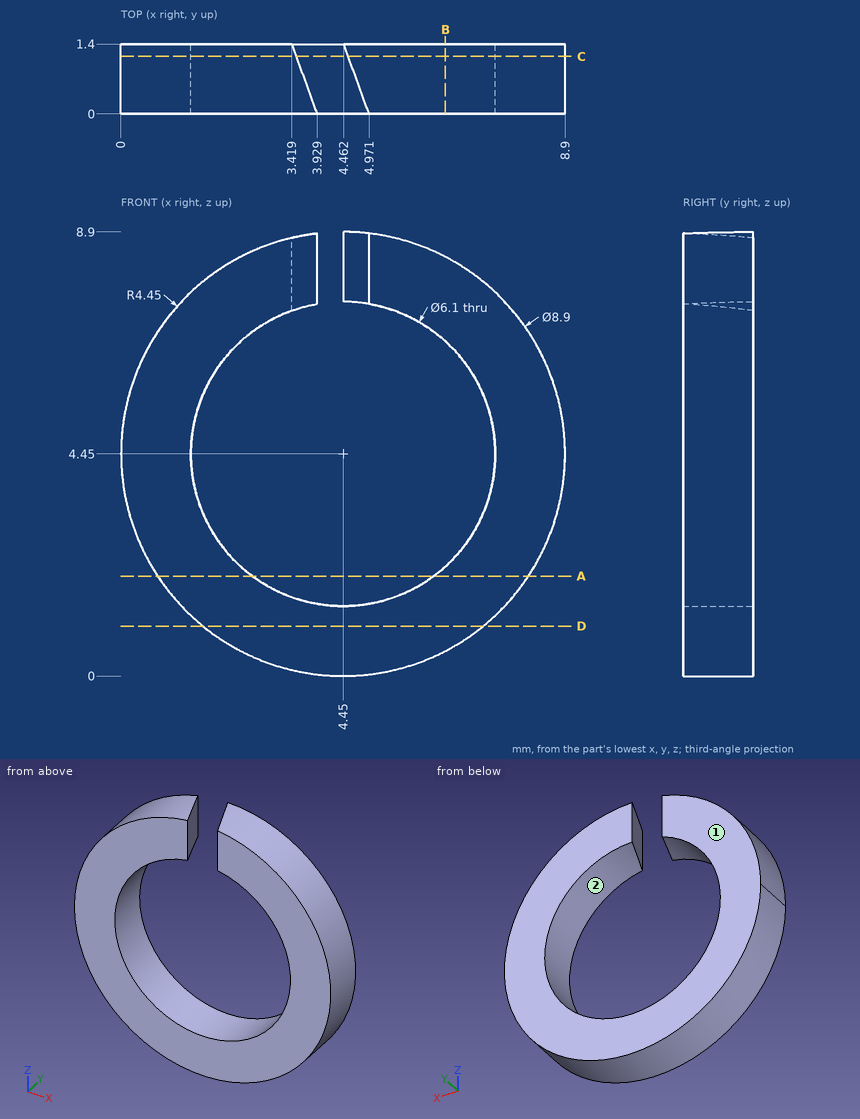
Design review of the part shown in the three views and the two pictorial views. Dimensions are in mm from the part's minimum x, y and z. Coordinates: 2 decimals unless noted, no trailing zeros. Order: outer loops, then holes, each group sorted by start corner. A loop starts at its lowest first (then second) coordinate and runs counter-clockwise, first axis right, second up.
1) Clearance check with flat-ended pins moving along their axes: pin 1 (3 mm diameter, centred on x = 8, z = 7.5, fed in from -Y); pin 2 (5 mm diameter, centred on x = 4.45, z = 4.45, fed in from -Y). State where each tip first meets the part, or that it passes through.
2) Mouldability with a two-part tool opening along X and no side actions: class the marked faces 1 and 2 as +X half, -X half, draft (parallel to the pull), parting line (faces both ways), or undercut.
3) Take a section at A-A, the plane z = 2. Give the boundary of the cut face in (x, y) (1 decimal).
4) Wall thickness on line 1 along X through (y, z) = (0.6, 4.5); line 2 along Z through (x, y) = (4.45, 1.05); line 3 along X through (y, z) = (1.3, 3.5): over which ranges is each line inside the solid? List them lowest first.
5) Take a section at C-C, the plane y = 1.15. Give the boundary of the cut face in (x, z).
6) Take a section at B-B, the plane x = 6.5. Give the boundary of the cut face in (y, z).
7) Take a section at D-D, the plane z = 1. Give the boundary of the cut face in (x, y).
Returned:
1. pin 1: stops at y = 0
1. pin 2: passes through
2. face 1: draft
2. face 2: undercut
3. outline: (0.7, 0) - (2.6, 0) - (2.6, 1.4) - (0.7, 1.4) - close; (6.3, 0) - (8.2, 0) - (8.2, 1.4) - (6.3, 1.4) - close
4. line 1: x = 0 to 1.4, 7.5 to 8.9
4. line 2: z = 0 to 1.4
4. line 3: x = 0.1 to 1.55, 7.35 to 8.8
5. outline: (3.51, 7.35) - (3.51, 8.8) arc R4.45 ccw (long way) to (4.55, 8.9) - (4.55, 7.5) arc R3.05 cw (long way) to start
6. outline: (0, 0.5) - (1.4, 0.5) - (1.4, 2.19) - (0, 2.19) - close; (0, 6.71) - (1.4, 6.71) - (1.4, 8.4) - (0, 8.4) - close
7. outline: (1.64, 0) - (7.26, 0) - (7.26, 1.4) - (1.64, 1.4) - close
